The model under review builds one solid part; all positions refer to its coordinate system, in mm. A direction names the side the tool comes from. Coordinates: 2 decimals unless noted, no trailing zeros. Write each loop counter-clockwise with the first axis right and the second up, starting at its lowest first coordinate (ties: lowest second). Pieces come first, ordered by that corner, then holes. Notation, with made-up numbers: (59.25, -37) - (82.25, -37) arc R9 cw to (82.25, -25) - close; hole circle Ø7 at (40.5, 63.25). An arc over 180 degrees is marked (long way). Put each result on its own line as item: value. Start each with the question number.
Item 1: To check wall thickness, follow L1, parallel to X at y = 11, z = 0; L2, parallel to X at y = 5.25, z = 0; L3, parallel to Y at x = 13.75, z = -1. State the ranges of each line that lie inside material, in increasing order. Write a range as [from, to].
Item 2: Mouldability with a two-part tool opening along Z and no side actions: class faces 1 (the face through (-13.18, 15.04, -2.93)), 2 (the face through (-12, 22.104, -7)), 3 (the face through (-14.49, 13.29, -3.22)) as pulls with the +Z half, pulls with the -Z half, needs draft (parallel to the pull), parting line crosses it, or undercut.
Item 3: Consider section B-B on y = 6.5. Give the boundary of the cut face in (x, z), then the cut area to 3 significant figures.
Item 4: For pin 1 (4 mm diameter, centred on x = 0.5, y = 3, fed in from -Z); pin 2 (5 mm diameter, centred on x = 11, z = 11, fed in from -Y); pin 3 (6 mm diameter, centred on x = -0.5, z = 6.5, fed in from -Y); pin 4 (5 mm diameter, centred on y = 9, z = -5, fed in from -X), all flat-tipped, find the tip position at first contact; note any pin that passes through.
Item 5: Consider section A-A on y = 19.75. Give the boundary of the cut face in (x, z).
Item 6: Machinability: for faces 4 (the face through (-1.9, 7.767, 12.1)), 5 (the face through (-10, 4.71, 10)), which of the approach directions +Z, -Z, +X, -X, +Y, -Y give a long, thin tool a straight path to every point of the face, cutting with its end or side? Answer none if there is none.
```python
from build123d import *


# Not quite as in the source:
# - ends of sketch curves that miss each other by under 0.0002 mm in the source are joined


with BuildPart() as f1:
    # F0 (on Right) → F1 (revolve)
    with BuildSketch(Plane.YZ):
        Polygon((0, 13.5986562818), (-0.5646626814, 12.0454436497), (7.7669508635, 12.0454436497), (7.7669508635, 13.5), (22.1037470661, 13.5), (22.1037470661, 14.8426934129), (4.7102691696, 14.8426934129), (4.7102691696, 13.7568386238), (4.6180134269, 12.6362909356), (4.1976161123, 13.6032054045), (4.0180134269, 12.6362909356), (3.5980134269, 13.6024472174), (3.4184107415, 12.6355327485), (2.9984107415, 13.6016890303), (2.8188080562, 12.6347745614), (2.3988080562, 13.6009308432), (2.2192053708, 12.6340163742), (1.7992053708, 13.6001726561), (1.6196026854, 12.6332581871), (1.1996026854, 13.5994144689), (1.02, 12.6325), (0.6, 13.5986562818), (0.4203973146, 12.6317418129), align=None)
    revolve(axis=Axis((0, 14.1517902564, 0), (0, 1, 0)))


solid = f1.part
```
Report:
1. L1: [-14.84, -13.5], [13.5, 14.84]
1. L2: [-14.84, -12.05], [12.05, 14.84]
1. L3: [4.71, 22.1]
2. face 1: undercut
2. face 2: needs draft
2. face 3: parting line crosses it
3. outline: circle Ø29.69 at (0, 0); hole circle Ø24.09 at (0, 0)
3. area: 236 mm²
4. pin 1: z = -14.84
4. pin 2: y = -0.2
4. pin 3: through
4. pin 4: x = -14.63
5. outline: circle Ø29.69 at (0, 0); hole circle Ø27 at (0, 0)
6. face 4: +Y
6. face 5: -Y
